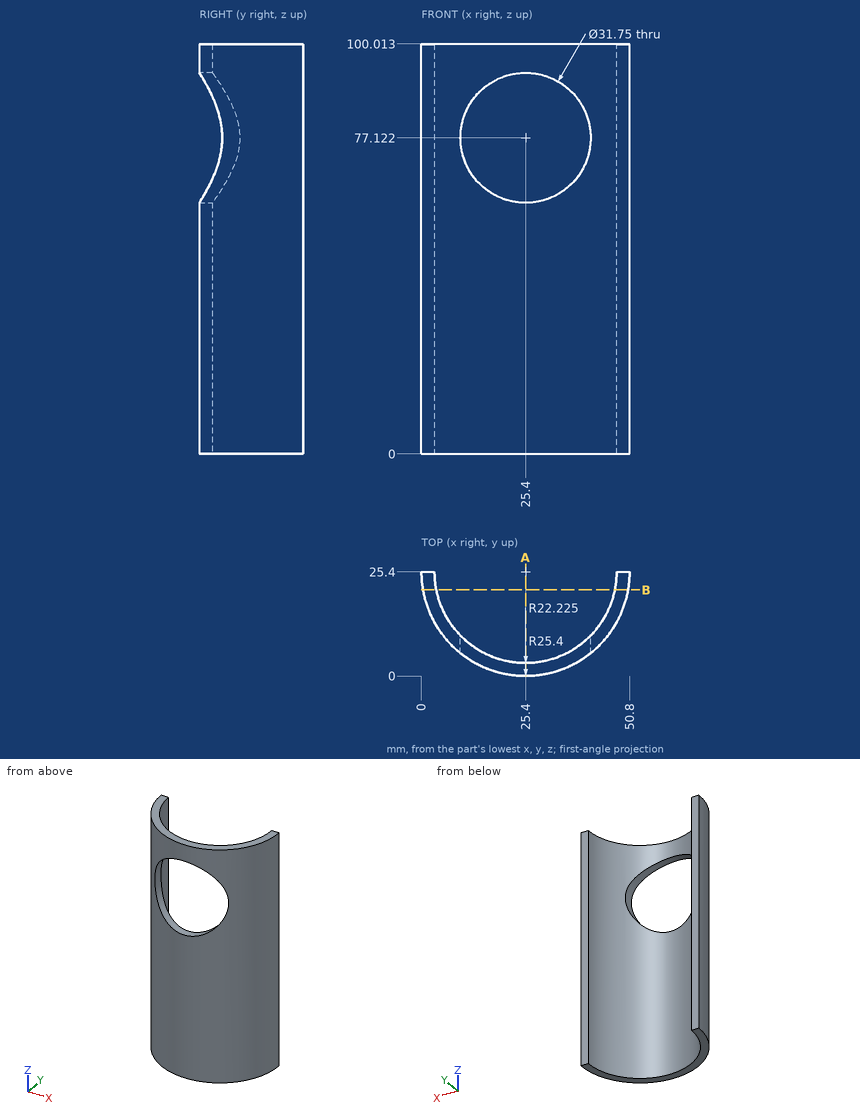
Check sheet for the drawn part. Datum: minimum x, y, z corner. Units: mm. Give positions to 0.01 mm unless a question says otherwise; leave off trailing zeros. Order: outer loops, then holes, each group sorted by start corner. A loop starts at its lowest first (then second) coordinate and runs counter-clockwise, first axis right, second up. Notation, with made-up numbers: (-10, -7) - (7, -7) arc R11 cw to (7, 4) - close; hole circle Ø11 at (-40, 6). An arc over 180 degrees is marked (long way). Answer as a JSON object with one key per item and string values.
(1) Material ranges on line 1 (X direction, y = 16.5, z = 42.5) (1 decimal); line 2 (X direction, y = 9.5, z = 51.5) (1 decimal); line 3 (Y direction, x = 25, z = 37.5), recorded low to high.
Report:
{"line 1": "1.6 to 5, 45.8 to 49.2", "line 2": "5.6 to 9.9, 40.9 to 45.2", "line 3": "0 to 3.18"}
(2) Depth check by flat-ended pin: pin 1 Ø8 at (y, z) = (6.5, 57) entering from +X; pin 2 Ø2 at (x, z) = (28.5, 42) entering from +Y; pin 3 Ø4 at (y, z) = (20, 48.5) entering from -X; pin 4 Ø12 at (x, y) = (10.5, 3) entering from -Z. Enter the tip coordinate at first touch or a pass-through.
Report:
{"pin 1": "x = 45.97", "pin 2": "y = 3.56", "pin 3": "x = 0.23", "pin 4": "z = 0"}
(3) Cross-section at A-A (x = 25.4). Record the cut outline in (y, z) (1 decimal), then the cut area to 3 significant figures.
Report:
{"outline": "(0, 0) - (3.2, 0) - (3.2, 61.2) - (0, 61.2) - close; (0, 93) - (3.2, 93) - (3.2, 100) - (0, 100) - close", "area": "217 mm^2"}
(4) Cross-section at B-B (y = 21). Record the cut outline in (x, z) (1 decimal).
Report:
{"outline": "(0.4, 0) - (3.6, 0) - (3.6, 100) - (0.4, 100) - close; (47.2, 0) - (50.4, 0) - (50.4, 100) - (47.2, 100) - close"}
